```python
from build123d import *

# Parameters (mm, degrees)
EXTRUDE_1_DEPTH     = 32
EXTRUDE_START       = 32
SKETCH_2_R          = 2.1
EXTRUDE_2_DEPTH     = 6
EXTRUDE_START_2     = -26
SKETCH_2_3_R        = 2.1
EXTRUDE_3_DEPTH     = 6
CUT_EXTRUDE_START   = 32
SKETCH_2_4_R        = 2.1
CUT_EXTRUDE_1_DEPTH = 4
CUT_EXTRUDE_START_2 = -28
SKETCH_2_5_R        = 2.1
CUT_EXTRUDE_2_DEPTH = 4
SKETCH_3_W          = 48.2
SKETCH_3_H          = 35
CUT_EXTRUDE_3_DEPTH = 0.8
SKETCH_4_W          = 41.9
SKETCH_4_H          = 32.8
CUT_EXTRUDE_4_DEPTH = 92.767243652
SKETCH_7_R          = 4
CUT_EXTRUDE_5_DEPTH = 10
SKETCH_8_R          = 2.55
EXTRUDE_4_DEPTH     = 2
SKETCH_9_R          = 1.4
CUT_EXTRUDE_6_DEPTH = 3
CHAMFER_1_SIZE      = 1.5


with BuildPart() as part:
    # Эскиз1 → Бобышка-Вытянуть1 (new, symmetric)
    with BuildSketch(Plane.XY):
        with BuildLine():
            Line((59.5, 80), (23.450862198, 80))
            ThreePointArc((23.450862198, 80), (19.977898644, 79.69615506), (16.610459331, 78.793852416))
            Line((16.610459331, 78.793852416), (-60.52606043, 50.718455248))
            ThreePointArc((-60.52606043, 50.718455248), (-61.326284287, 50.279437406), (-61.957456133, 49.620106694))
            Line((-61.957456133, 49.620106694), (-59.5, 47.899377385))
            Line((-59.5, 47.899377385), (17.636519761, 75.974774553))
            ThreePointArc((17.636519761, 75.974774553), (20.498843177, 76.741731801), (23.450862198, 77))
            Line((23.450862198, 77), (59.5, 77))
            Line((59.5, 77), (61.621320344, 79.121320344))
            ThreePointArc((61.621320344, 79.121320344), (60.648050297, 79.771638598), (59.5, 80))
        make_face()
    extrude(amount=EXTRUDE_1_DEPTH, both=True)

    # Эскиз2 → Бобышка-Вытянуть2 (add)
    # profile 1 of 4: a face of its own
    with BuildSketch(Plane.XY.offset(EXTRUDE_START)):
        with BuildLine():
            Line((51.3, 80), (51.3, 74.9))
            ThreePointArc((51.3, 74.9), (55.4, 70.8), (59.5, 74.9))
            Line((59.5, 74.9), (59.5, 80))
            Line((59.5, 80), (51.3, 80))
        make_face()
        with Locations((55.4, 74.9)):
            Circle(SKETCH_2_R, mode=Mode.SUBTRACT)
    # profile 2 of 4: a face of its own
    with BuildSketch(Plane.XY.offset(EXTRUDE_START)):
        with Locations((55.4, 74.9)):
            Circle(SKETCH_2_R)
    # profile 3 of 4: a face of its own
    with BuildSketch(Plane.XY.offset(EXTRUDE_START)):
        with BuildLine():
            ThreePointArc((-51.3, 47.156882024), (-55.4, 43.056882024), (-59.5, 47.156882024))
            Line((-59.5, 47.156882024), (-59.5, 51.091910703))
            Line((-59.5, 51.091910703), (-51.3, 54.076466624))
            Line((-51.3, 54.076466624), (-51.3, 47.156882024))
        make_face()
        with Locations((-55.4, 47.156882024)):
            Circle(SKETCH_2_R, mode=Mode.SUBTRACT)
    # profile 4 of 4: a face of its own
    with BuildSketch(Plane.XY.offset(EXTRUDE_START)):
        with Locations((-55.4, 47.156882024)):
            Circle(SKETCH_2_R)
    extrude(amount=-EXTRUDE_2_DEPTH)

    # Эскиз2<3> → Бобышка-Вытянуть3 (add)
    # profile 1 of 4: a face of its own
    with BuildSketch(Plane.XY.offset(EXTRUDE_START_2)):
        with BuildLine():
            Line((51.3, 80), (51.3, 74.9))
            ThreePointArc((51.3, 74.9), (55.4, 70.8), (59.5, 74.9))
            Line((59.5, 74.9), (59.5, 80))
            Line((59.5, 80), (51.3, 80))
        make_face()
        with Locations((55.4, 74.9)):
            Circle(SKETCH_2_3_R, mode=Mode.SUBTRACT)
    # profile 2 of 4: a face of its own
    with BuildSketch(Plane.XY.offset(EXTRUDE_START_2)):
        with Locations((55.4, 74.9)):
            Circle(SKETCH_2_3_R)
    # profile 3 of 4: a face of its own
    with BuildSketch(Plane.XY.offset(EXTRUDE_START_2)):
        with BuildLine():
            ThreePointArc((-51.3, 47.156882024), (-55.4, 43.056882024), (-59.5, 47.156882024))
            Line((-59.5, 47.156882024), (-59.5, 51.091910703))
            Line((-59.5, 51.091910703), (-51.3, 54.076466624))
            Line((-51.3, 54.076466624), (-51.3, 47.156882024))
        make_face()
        with Locations((-55.4, 47.156882024)):
            Circle(SKETCH_2_3_R, mode=Mode.SUBTRACT)
    # profile 4 of 4: a face of its own
    with BuildSketch(Plane.XY.offset(EXTRUDE_START_2)):
        with Locations((-55.4, 47.156882024)):
            Circle(SKETCH_2_3_R)
    extrude(amount=-EXTRUDE_3_DEPTH)

    # Эскиз2<4> → Вырез-Вытянуть1 (cut)
    with BuildSketch(Plane.XY.offset(CUT_EXTRUDE_START)):
        with Locations((55.4, 74.9)):
            Circle(SKETCH_2_4_R)
        with Locations((-55.4, 47.156882024)):
            Circle(SKETCH_2_4_R)
    extrude(amount=-CUT_EXTRUDE_1_DEPTH, mode=Mode.SUBTRACT)

    # Эскиз2<5> → Вырез-Вытянуть2 (cut)
    with BuildSketch(Plane.XY.offset(CUT_EXTRUDE_START_2)):
        with Locations((55.4, 74.9)):
            Circle(SKETCH_2_5_R)
        with Locations((-55.4, 47.156882024)):
            Circle(SKETCH_2_5_R)
    extrude(amount=-CUT_EXTRUDE_2_DEPTH, mode=Mode.SUBTRACT)

    # Эскиз3 → Вырез-Вытянуть3 (cut)
    with BuildSketch(Plane(origin=(-22.354740965, 61.419146018, 0), x_dir=(0.9396926207859082, 0.3420201433256692, 0), z_dir=(0.3420201433256692, -0.9396926207859082, 0))):
        with Locations((14.320840982, 0)):
            Rectangle(SKETCH_3_W, SKETCH_3_H)
    extrude(amount=-CUT_EXTRUDE_3_DEPTH, mode=Mode.SUBTRACT)

    # Эскиз4 → Вырез-Вытянуть4 (cut, through all)
    with BuildSketch(Plane(origin=(-22.354740965, 61.419146018, 0), x_dir=(0.9396926207859082, 0.3420201433256692, 0), z_dir=(0.3420201433256692, -0.9396926207859082, 0))):
        with Locations((16.370840982, 0)):
            Rectangle(SKETCH_4_W, SKETCH_4_H)
    extrude(amount=-CUT_EXTRUDE_4_DEPTH, mode=Mode.SUBTRACT)

    # Эскиз7 → Вырез-Вытянуть5 (cut)
    with BuildSketch(Plane(origin=(-23.380801395, 64.238223881, 0), x_dir=(0.9396926207859081, 0.34202014332566955, 0), z_dir=(-0.34202014332566955, 0.9396926207859082, 0))):
        with Locations(Location((-24.429159018, 10.25, 0), (0, 0, 180))):
            Circle(SKETCH_7_R)
        with Locations(Location((-24.414159018, -3.75, 0), (0, 0, 180))):
            Circle(SKETCH_7_R)
        with Locations(Location((-24.414159018, -15.75, 0), (0, 0, 180))):
            Circle(SKETCH_7_R)
    extrude(amount=-CUT_EXTRUDE_5_DEPTH, mode=Mode.SUBTRACT)

    # Эскиз8 → Бобышка-Вытянуть4 (add)
    with BuildSketch(Plane(origin=(-22.354740965, 61.419146018, 0), x_dir=(0.9396926207859081, 0.3420201433256697, 0), z_dir=(0.34202014332566966, -0.939692620785908, 0))):
        with Locations(Location((40.970840982, 15, 0), (0, 0, 180))):
            Circle(SKETCH_8_R)
        with Locations(Location((40.970840982, -15, 0), (0, 0, 180))):
            Circle(SKETCH_8_R)
        with Locations(Location((-36.029159018, -16.5, 0), (0, 0, 180))):
            Circle(SKETCH_8_R)
        with Locations(Location((-36.029159018, 16.5, 0), (0, 0, 180))):
            Circle(SKETCH_8_R)
    extrude(amount=EXTRUDE_4_DEPTH)

    # Эскиз9 → Вырез-Вытянуть6 (cut)
    with BuildSketch(Plane(origin=(-21.670700678, 59.539760777, 0), x_dir=(0.9396926207859104, 0.34202014332566316, 0), z_dir=(0.34202014332566316, -0.9396926207859104, 0))):
        with Locations((40.970840982, -15)):
            Circle(SKETCH_9_R)
        with Locations((40.970840982, 15)):
            Circle(SKETCH_9_R)
        with Locations((-36.029159018, -16.5)):
            Circle(SKETCH_9_R)
        with Locations((-36.029159018, 16.5)):
            Circle(SKETCH_9_R)
    extrude(amount=-CUT_EXTRUDE_6_DEPTH, mode=Mode.SUBTRACT)

    # Фаска1
    chamfer_1_edges = [part.edges().sort_by_distance(p)[0] for p in [
        (-27.683803334, 62.672059257, 0),
        (-7.997242928, 69.83738126, 16.4),
        (11.689317477, 77.002703262, 0),
        (-7.997242928, 69.83738126, -16.4),
    ]]
    chamfer(chamfer_1_edges, length=CHAMFER_1_SIZE)


solid = part.part
```
CAD build for the part. Positions are in the model's coordinates, mm. A direction names the side the tool comes from. Give positions to 0.01 mm unless a question says otherwise; leave off trailing zeros. Write each loop counter-clockwise with the first axis right and the second up, starting at its lowest first coordinate (ties: lowest second). Pieces come first, ordered by that corner, then holes. Notation, with made-up numbers: (-34.75, 58.25) -> (-21.75, 58.25) arc R17 cw to (-21.75, 66.25) -> close; hole circle Ø6 at (20, 85.5). An arc over 180 degrees is marked (long way). Write each question's results on one line, items separated by ' | '.
1. Wall check: probe 1 along Z at (x, y) = (-45, 54); probe 2 along Y at (x, z) = (55.4, -28.8); probe 3 along Z at (x, y) = (-47, 53.5). Give the ranges that are in metal, low to high. Write a range as [from, to].
Geometry check:
probe 1: [-32, -14.2], [-6.3, -0.21], [7.71, 11.79], [19.71, 32] | probe 2: [70.8, 72.8], [77, 80] | probe 3: [-32, -13.98], [-6.52, 0.02], [7.48, 12.02], [19.48, 32]
2. Two-plate mould, pull along Y, no slides. Class faces 1 (the flat face through (-56.57, 50.03, 16.52)), 2 (the flat face through (42, 80, 0)), 3 (the cylindrical face through (-45.002, 54.795, -0.155)), 4 (the flat face through (-60.746, 48.772, 0.448)): pulls with the +Y half, pulls with the -Y half, needs draft (parallel to the pull), parting line crosses it, or undercut.
Geometry check:
face 1: undercut | face 2: pulls with the +Y half | face 3: parting line crosses it | face 4: pulls with the -Y half
3. Cut at C-C, the plane x = 55.4. Write the cut outline in (y, z), then the cut area to 3 significant figures.
Geometry check:
outline: (70.8, -32) -> (72.8, -32) -> (72.8, -28) -> (77, -28) -> (77, -32) -> (80, -32) -> (80, 32) -> (77, 32) -> (77, 28) -> (72.8, 28) -> (72.8, 32) -> (70.8, 32) -> (70.8, 26) -> (77, 26) -> (77, -26) -> (70.8, -26) -> close | area: 233 mm²
4. Cut at D-D, the plane x = 0.5. Write the cut outline in (y, z), then the cut area to 3 significant figures.
Geometry check:
outline: (69.74, -32) -> (72.93, -32) -> (72.93, -17.9) -> (71.33, -16.4) -> (70.59, -16.4) -> (70.59, -17.5) -> (69.74, -17.5) -> close; (69.74, 17.5) -> (70.59, 17.5) -> (70.59, 16.4) -> (71.33, 16.4) -> (72.93, 17.9) -> (72.93, 32) -> (69.74, 32) -> close | area: 95.3 mm²
5. Cut at A-A, the plane z = 9.5. Write the cut outline in (x, y), then the cut area to 3 significant figures.
Geometry check:
outline: (-61.96, 49.62) -> (-59.5, 47.9) -> (-31.54, 58.07) -> (-31.82, 58.83) -> (-26.93, 60.6) -> (-27.17, 61.26) -> (-29.09, 62.16) -> (-60.53, 50.72) arc R3 ccw to start; (12.2, 75.59) -> (12.44, 74.94) -> (13.48, 75.31) -> (13.75, 74.56) -> (17.64, 75.97) arc R17 cw to (23.45, 77) -> (59.5, 77) -> (61.62, 79.12) arc R3 ccw to (59.5, 80) -> (23.45, 80) arc R20 ccw to (16.61, 78.79) -> (13.1, 77.52) -> close | area: 247 mm²
6. Cut at B-B, the plane y = 67. Write the cut outline in (x, z).
Geometry check:
outline: (-15.79, -32) -> (-7.02, -32) -> (-7.02, -17.5) -> (-9.36, -17.5) -> (-9.36, -16.4) -> (-11.41, -16.4) -> (-15.79, -17.9) -> close; (-15.79, 17.9) -> (-11.41, 16.4) -> (-9.36, 16.4) -> (-9.36, 17.5) -> (-7.02, 17.5) -> (-7.02, 32) -> (-15.79, 32) -> close
7. Which spindle directions (+Z, -Z, +X, -X, +Y, -Y) get a long thin tool onto all of the face, cutting with end or side? Do faces 5 (the flat face through (-51.3, 49, -29)), 6 (the cylindrical face through (57.403, 75.531, 30.028)), 7 (the flat face through (-55, 47, -28)). Say none if no direction does.
Geometry check:
face 5: +Z, -Z, +X, -Y | face 6: +Z | face 7: -Z
8. Drop flat-ended pins along their axis: P1, Ø0.6, axis at y = 47.5, z = -29.5, coming from the -X side; P2, Ø12, axis at x = 18, z = 9, coming from the -Y side; P3, Ø1, axis at x = -42, z = -15, coming from the +Y side. Give the stop position or say it passes through.
Geometry check:
P1: x = -59.5 | P2: y = 72.75 | P3: y = 57.64
